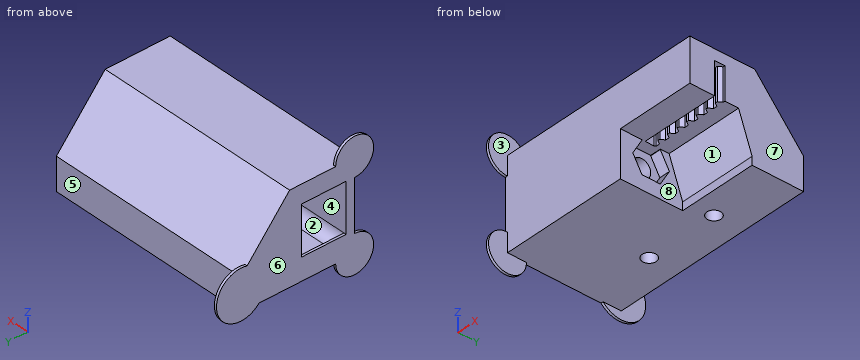
from build123d import *

# Parameters (mm, degrees)
SKETCH1_W           = 38.5
SKETCH1_H           = 21
BOSS_EXTRUDE1_DEPTH = 16.5
SKETCH2_R           = 1.7
CUT_EXTRUDE1_DEPTH  = 38.5
SKETCH2_5_R         = 1.7
SKETCH2_5_W         = 0.075
SKETCH2_5_H         = 3.377499074
SKETCH2_5_W_2       = 1.5
SKETCH2_5_H_2       = 4
CUT_EXTRUDE2_DEPTH  = 14.5
CUT_EXTRUDE3_START  = -16.5
SKETCH2_6_R         = 1.7
SKETCH2_6_W         = 0.075
SKETCH2_6_H         = 3.377499074
CUT_EXTRUDE3_DEPTH  = 2
CUT_EXTRUDE4_DEPTH  = 18
SKETCH4_R           = 1.3
CUT_EXTRUDE5_DEPTH  = 9.5
CUT_EXTRUDE7_DEPTH  = 6
CHAMFER3_SIZE       = 1
BOSS_EXTRUDE2_DEPTH = 0.44


with BuildPart() as part:
    # Sketch1 → Boss-Extrude1 (new body)
    with BuildSketch(Plane.XY):
        Rectangle(SKETCH1_W, SKETCH1_H)
    extrude(amount=BOSS_EXTRUDE1_DEPTH)

    # Sketch2 → Cut-Extrude1 (cut)
    with BuildSketch(Plane(origin=(19.25, 0, 0), x_dir=(0, 0, -1), z_dir=(1, 0, 0))):
        Polygon((-16.5, 10.5), (-16.5, 1.5), (-6, 10.5), align=None)
        with Locations((-5.5, -4.82)):
            Circle(SKETCH2_R)
    extrude(amount=-CUT_EXTRUDE1_DEPTH, mode=Mode.SUBTRACT)

    # Sketch2<5> → Cut-Extrude2 (cut)
    with BuildSketch(Plane(origin=(19.25, 0, 0), x_dir=(0, 0, -1), z_dir=(1, 0, 0))):
        Polygon((-8.5, -6.508749537), (-8.5, -10.5), (-1.5, -10.5), (-1.5, -6.5), (0, -6.5), (0, 1), (-1.5, 1), (-8.5, -1.5), (-8.5, -3.131250463), (-8.425, -3.131250463), (-5.5, -1.442500925), (-2.575, -3.131250463), (-2.575, -6.508749537), (-5.5, -8.197499075), (-8.425, -6.508749537), align=None)
        Polygon((-8.425, -6.508749537), (-5.5, -8.197499075), (-2.575, -6.508749537), (-2.575, -3.131250463), (-5.5, -1.442500925), (-8.425, -3.131250463), align=None)
        with Locations((-5.5, -4.82)):
            Circle(SKETCH2_5_R, mode=Mode.SUBTRACT)
        with Locations((-8.4625, -4.82)):
            Rectangle(SKETCH2_5_W, SKETCH2_5_H)
        with Locations((-0.75, -8.5)):
            Rectangle(SKETCH2_5_W_2, SKETCH2_5_H_2)
    extrude(amount=-CUT_EXTRUDE2_DEPTH, mode=Mode.SUBTRACT)

    # Sketch2<6> → Cut-Extrude3 (cut)
    with BuildSketch(Plane(origin=(19.25, 0, 0), x_dir=(0, 0, -1), z_dir=(1, 0, 0)).offset(CUT_EXTRUDE3_START)):
        Polygon((-8.425, -6.508749537), (-5.5, -8.197499075), (-2.575, -6.508749537), (-2.575, -3.131250463), (-5.5, -1.442500925), (-8.425, -3.131250463), align=None)
        with Locations((-5.5, -4.82)):
            Circle(SKETCH2_6_R, mode=Mode.SUBTRACT)
        with Locations((-5.5, -4.82)):
            Circle(SKETCH2_6_R)
        with Locations((-8.4625, -4.82)):
            Rectangle(SKETCH2_6_W, SKETCH2_6_H)
    extrude(amount=CUT_EXTRUDE3_DEPTH, mode=Mode.SUBTRACT)

    # Sketch3 → Cut-Extrude4 (cut)
    with BuildSketch(Plane.ZY.offset(19.25)):
        with BuildLine():
            Line((13.1, -8.92), (4.1, -8.92))
            ThreePointArc((4.1, -8.92), (2.685786438, -8.334213562), (2.1, -6.92))
            Line((2.1, -6.92), (2.1, -2.72))
            ThreePointArc((2.1, -2.72), (2.685786438, -1.305786438), (4.1, -0.72))
            Line((4.1, -0.72), (13.1, -0.72))
            ThreePointArc((13.1, -0.72), (14.514213562, -1.305786438), (15.1, -2.72))
            Line((15.1, -2.72), (15.1, -6.92))
            ThreePointArc((15.1, -6.92), (14.514213562, -8.334213562), (13.1, -8.92))
        make_face()
    extrude(amount=-CUT_EXTRUDE4_DEPTH, mode=Mode.SUBTRACT)

    # Sketch4 → Cut-Extrude5 (cut)
    with BuildSketch(Plane(origin=(0, 0, 0), x_dir=(-1, 0, 0), z_dir=(0, 0, -1))):
        with Locations((-6.75, 5)):
            Circle(SKETCH4_R)
        with Locations((6.75, 5)):
            Circle(SKETCH4_R)
    extrude(amount=-CUT_EXTRUDE5_DEPTH, mode=Mode.SUBTRACT)

    # Sketch5 → Cut-Extrude7 (cut)
    with BuildSketch(Plane(origin=(0, 0, 8.5), x_dir=(-1, 0, 0), z_dir=(0, 0, -1))):
        Polygon((-20.249996698, -5.92), (-4.75, -5.92), (-4.75, -4.253375074), (-4.90002704, -4.02), (-5.600019193, -4.02), (-6.050019814, -4.72), (-6.250019814, -4.72), (-6.450023117, -4.72), (-6.900023738, -4.02), (-7.600015891, -4.02), (-8.050016512, -4.72), (-8.250016512, -4.72), (-8.450019814, -4.72), (-8.900020436, -4.02), (-9.600012588, -4.02), (-10.05001321, -4.72), (-10.25001321, -4.72), (-10.450016512, -4.72), (-10.900017133, -4.02), (-11.600009286, -4.02), (-12.050009907, -4.72), (-12.250009907, -4.72), (-12.45001321, -4.72), (-12.900013831, -4.02), (-13.600005984, -4.02), (-14.050006605, -4.72), (-14.250006605, -4.72), (-14.450009907, -4.72), (-14.900010528, -4.02), (-15.600002681, -4.02), (-16.050003302, -4.72), (-16.250003302, -4.72), (-16.450006605, -4.72), (-16.900007226, -4.02), (-17.599999379, -4.02), (-18.05, -4.72), (-18.250003302, -4.72), (-18.450003302, -4.72), (-18.900003924, -4.02), (-19.599996076, -4.02), (-20.049996698, -4.72), (-20.249996698, -4.72), align=None)
    extrude(amount=-CUT_EXTRUDE7_DEPTH, mode=Mode.SUBTRACT)

    # Chamfer3
    chamfer3_edges = [part.edges().sort_by_distance(p)[0] for p in [
        (8.05, 5, 9.5),
        (-5.45, 5, 9.5),
    ]]
    chamfer(chamfer3_edges, length=CHAMFER3_SIZE)

    # Sketch6 → Boss-Extrude2 (add)
    with BuildSketch(Plane.ZY.offset(19.25)):
        with BuildLine():
            Line((4.1, -8.92), (4.1, -0.72))
            ThreePointArc((4.1, -0.72), (2.685786438, -1.305786438), (2.1, -2.72))
            Line((2.1, -2.72), (2.1, -6.92))
            ThreePointArc((2.1, -6.92), (2.685786438, -8.334213562), (4.1, -8.92))
        make_face()
        with BuildLine():
            ThreePointArc((15.1, -2.72), (14.514213562, -1.305786438), (13.1, -0.72))
            Line((13.1, -0.72), (13.1, -8.92))
            ThreePointArc((13.1, -8.92), (14.514213562, -8.334213562), (15.1, -6.92))
            Line((15.1, -6.92), (15.1, -2.72))
        make_face()
        with BuildLine():
            Line((16.5, -10.5), (13, -10.5))
            ThreePointArc((13, -10.5), (18.974873734, -12.974873734), (16.5, -7))
            Line((16.5, -7), (16.5, -10.5))
        make_face()
        with BuildLine():
            ThreePointArc((0, -7), (-2.474873734, -12.974873734), (3.5, -10.5))
            Line((3.5, -10.5), (0, -10.5))
            Line((0, -10.5), (0, -7))
        make_face()
        with BuildLine():
            ThreePointArc((7.348925314, 9.343778302), (1.710593433, 14.811314267), (0, 7.145898034))
            Line((0, 7.145898034), (0, 10.5))
            Line((0, 10.5), (6, 10.5))
            Line((6, 10.5), (7.348925314, 9.343778302))
        make_face()
    extrude(amount=-BOSS_EXTRUDE2_DEPTH)


solid = part.part
The model under review builds one solid part; all positions refer to its coordinate system, in mm. Face numbers are marked on the shaded views. A direction names the side the tool comes from. Give positions to 0.01 mm unless a question says otherwise; leave off trailing zeros. Write each loop counter-clockwise with the first axis right and the second up, starting at its lowest first coordinate (ties: lowest second). Pieces come first, ordered by that corner, then holes.
1. Draft analysis for pull direction Y (two halves, no side actions). For the marked faces 1, 2 and 3, state which applies: +Y half, -Y half, draft (parallel to the pull), parting line (faces both ways), or undercut.
2. Tool access review of the marked faces 4, 5, 6, 7 and 8: name each direction out of +Z, -Z, +X, -X, +Y, -Y from which nothing blocks a thin tool from reaching the whole face with its end or side.
3. Add section B-B, the plane x = -10. Write out the cut boundary in (y, z).
4. Add section A-A, the plane x = 1.5. Write out the cut boundary in (y, z).
5. For P1, Ø4, axis at x = -6.75, y = 5, coming from the -Z side; P2, Ø4, axis at x = -5.5, z = 14.5, coming from the +Y side; P3, Ø1.2, axis at x = 10, z = 1, coming from the -Y side, all flat-tipped, find the tip position at first contact; note any pin that passes through.
6. Wall thickness on L1, parallel to Y at x = -6.75, z = 6; L2, parallel to Y at x = 0.9, z = 5.5; L3, parallel to X at y = 4.75, z = 2.25: over which ranges is each line inside the solid? List them lowest first.
Worked answers:
1. face 1: -Y half
1. face 2: undercut
1. face 3: draft
2. face 4: -X
2. face 5: +Z, -Z, +X, +Y
2. face 6: +Z, -Z, -X, +Y, -Y
2. face 7: +Z, -Z, +X, +Y, -Y
2. face 8: -Z, +X, -Y
3. outline: (-10.5, 0) - (10.5, 0) - (10.5, 6) - (1.5, 16.5) - (-10.5, 16.5) - close; hole (-8.92, 4.1) arc R2 ccw to (-6.92, 2.1) - (-2.72, 2.1) arc R2 ccw to (-0.72, 4.1) - (-0.72, 13.1) arc R2 ccw to (-2.72, 15.1) - (-6.92, 15.1) arc R2 ccw to (-8.92, 13.1) - close
4. outline: (-10.5, 0) - (10.5, 0) - (10.5, 6) - (1.5, 16.5) - (-10.5, 16.5) - close; hole circle Ø3.4 at (-4.82, 5.5)
5. P1: stops at z = 0
5. P2: stops at y = 4.93
5. P3: stops at y = 0.96
6. L1: y = -10.5 to -8.92, -0.72 to 3.7, 6.3 to 10.5
6. L2: y = -10.5 to -6.52, -3.12 to 10.5
6. L3: x = -19.25 to -8.03, -5.47 to 5.47, 8.03 to 19.25
